from build123d import *

# Parameters (mm, degrees)
BOSS_EXTRUDE1_DEPTH = 12
SKETCH2_3_R         = 20
SKETCH2_3_R_2       = 9
BOSS_EXTRUDE2_DEPTH = 24
SKETCH2_4_R         = 27.5
SKETCH2_4_R_2       = 15
BOSS_EXTRUDE3_DEPTH = 18
BOSS_EXTRUDE4_DEPTH = 85
FILLET1_R           = 25


with BuildPart() as part:
    # Sketch2 → Boss-Extrude1 (new body)
    with BuildSketch(Plane.XY):
        with BuildLine():
            Line((-90, -100), (0, -100))
            Line((0, -100), (50, -100))
            Line((50, -100), (26.866088482, 5.870544241))
            ThreePointArc((26.866088482, 5.870544241), (27.341062829, 2.952335241), (27.5, 0))
            ThreePointArc((27.5, 0), (0, -27.5), (-27.5, 0))
            Line((-27.5, 0), (-27.5, -42))
            Line((-27.5, -42), (-70, -42))
            ThreePointArc((-70, -42), (-55.857864376, -47.857864376), (-50, -62))
            ThreePointArc((-50, -62), (-70, -82), (-90, -62))
            Line((-90, -62), (-90, -100))
        make_face()
    extrude(amount=BOSS_EXTRUDE1_DEPTH)

    # Sketch2_3 → Boss-Extrude2 (add)
    with BuildSketch(Plane.XY):
        with Locations(Location((-70, -62, 0), (0, 0, 180))):
            Circle(SKETCH2_3_R)
        with Locations((-70, -62)):
            Circle(SKETCH2_3_R_2, mode=Mode.SUBTRACT)
    extrude(amount=BOSS_EXTRUDE2_DEPTH)

    # Sketch2_4 → Boss-Extrude3 (add, symmetric)
    with BuildSketch(Plane.XY):
        Circle(SKETCH2_4_R)
        Circle(SKETCH2_4_R_2, mode=Mode.SUBTRACT)
    extrude(amount=BOSS_EXTRUDE3_DEPTH, both=True)

    # Sketch2_5 → Boss-Extrude4 (add)
    with BuildSketch(Plane.XY):
        Polygon((-90, -100), (0, -100), (50, -100), (50, -118), (-90, -118), align=None)
    extrude(amount=BOSS_EXTRUDE4_DEPTH)

    # Fillet1
    fillet1_edges = [part.edges().sort_by_distance(p)[0] for p in [
        (-27.5, -42, 6),
    ]]
    fillet(fillet1_edges, radius=FILLET1_R)


solid = part.part
Verification items for the finished model (mm, model axes). A direction names the side the tool comes from. Round coordinates to 2 decimals unless told otherwise and drop trailing zeros. Order: outer loops, then holes, each group sorted by start corner. A loop starts at its lowest first (then second) coordinate and runs counter-clockwise, first axis right, second up.
1. Go/stop test with flat-tipped pins: P1, Ø3, axis at x = 34, y = -99.5, coming from the -Z side; P2, Ø16.5, axis at x = 12, y = -2, coming from the +Z side; P3, Ø6, axis at y = -7, z = 7, coming from the -X side. Record where each tip stops, or that it passes through.
Final values:
P1: stops at z = 0
P2: stops at z = 18
P3: stops at x = -27.5
2. Section check B-B on y = -7. Record the cut outline in (x, z), then the cut area to 3 significant figures.
Final values:
outline: (-27.5, 0) - (-26.59, 0) - (-26.59, -18) - (-13.27, -18) - (-13.27, 18) - (-26.59, 18) - (-26.59, 12) - (-27.5, 12) - close; (13.27, -18) - (26.59, -18) - (26.59, 0) - (29.68, 0) - (29.68, 12) - (26.59, 12) - (26.59, 18) - (13.27, 18) - close
area: 1,010 mm2
3. Section check D-D on x = -64. Record the cut outline in (y, z).
Final values:
outline: (-118, 0) - (-68.71, 0) - (-68.71, 24) - (-81.08, 24) - (-81.08, 12) - (-100, 12) - (-100, 85) - (-118, 85) - close; (-55.29, 0) - (-42, 0) - (-42, 12) - (-42.92, 12) - (-42.92, 24) - (-55.29, 24) - close
4. Access from +Z, -Z, +X, -X, +Y, -Y to the whole of each face (thin tool, end or side, straight path). Record for faces 1 (the flat face through (-74, -53, 24)), 2 (the cylindrical face through (-88.475, -54.34, 17.165)), 3 (the flat face through (-27.5, -8, 6)).
Final values:
face 1: +Z, +X, -X, +Y
face 2: +Z
face 3: +Z, -Z, -X, +Y
5. Release check for a two-part mould opening along Y. For faces 4 (the flat face through (-19, -69, 0)), 5 (the cylindrical face through (-61.686, -65.447, 11.832)), 6 (the cylindrical face through (-14.985, 0.66, -0.252)), 7 (the flat face through (38.595, -47.806, 5.916)) record: +Y half, -Y half, draft (parallel to the pull), parting line (faces both ways), or undercut.
Final values:
face 4: draft
face 5: undercut
face 6: undercut
face 7: +Y half
6. Section check A-A on x = 0. Record the cut outline in (y, z), then the cut area to 3 significant figures.
Final values:
outline: (-118, 0) - (-27.5, 0) - (-27.5, -18) - (-15, -18) - (-15, 18) - (-27.5, 18) - (-27.5, 12) - (-100, 12) - (-100, 85) - (-118, 85) - close; (15, -18) - (27.5, -18) - (27.5, 18) - (15, 18) - close
area: 3,300 mm2
7. Section check C-C on z = -6. Record the cut outline in (x, y), then the cut area to 3 significant figures.
Final values:
outline: circle Ø55 at (0, 0); hole circle Ø30 at (0, 0)
area: 1,670 mm2
8. Thickness scan on L1, parallel to Y at x = -70, z = 14.25; L2, parallel to Y at x = -70, z = 11.5; L3, parallel to Z at x = -22, y = -22.5. Record the ranges inside material, lowest first.
Final values:
L1: y = -118 to -100, -82 to -71, -53 to -42
L2: y = -118 to -71, -53 to -42
L3: z = 0 to 12
